```python
from build123d import *

# Parameters (mm, degrees)
SKETCH1_R           = 7.5
BOSS_EXTRUDE1_DEPTH = 56
CUT_EXTRUDE1_DEPTH  = 38
SKETCH3_R           = 7
CUT_EXTRUDE2_DEPTH  = 26


with BuildPart() as part:
    # Sketch1 → Boss-Extrude1 (new body)
    with BuildSketch(Plane.XY):
        with BuildLine():
            Line((-28, -19), (31, -19))
            Line((31, -19), (46, -10.339745962))
            Line((46, -10.339745962), (46, 10.339745962))
            Line((46, 10.339745962), (31, 19))
            Line((31, 19), (6.698703146, 19))
            ThreePointArc((6.698703146, 19), (-12.009583788, 15.368092477), (-28, 5))
            Line((-28, 5), (-28, -19))
        make_face()
        Circle(SKETCH1_R, mode=Mode.SUBTRACT)
    extrude(amount=BOSS_EXTRUDE1_DEPTH)

    # Sketch2 → Cut-Extrude1 (cut)
    with BuildSketch(Plane(origin=(0, 19, 0), x_dir=(1, 0, 0), z_dir=(0, 1, 0))):
        Polygon((31, 0), (46, -15), (46, 0), align=None)
        Polygon((31, -56), (46, -41), (46, -56), align=None)
        Polygon((-28, -8), (-12, -8), (-12, -14), (20, -14), (20, -42), (-12, -42), (-12, -48), (-28, -48), align=None)
    extrude(amount=-CUT_EXTRUDE1_DEPTH, mode=Mode.SUBTRACT)

    # Sketch3 → Cut-Extrude2 (cut)
    with BuildSketch(Plane(origin=(46, 0, 0), x_dir=(0, 0, -1), z_dir=(1, 0, 0))):
        with Locations((-28, 0)):
            Circle(SKETCH3_R)
    extrude(amount=-CUT_EXTRUDE2_DEPTH, mode=Mode.SUBTRACT)


solid = part.part
```
Check sheet for the modelled part. Datum: model origin and axes. Units: mm. A direction names the side the tool comes from. Give positions to 0.01 mm unless a question says otherwise; leave off trailing zeros. Order: outer loops, then holes, each group sorted by start corner. A loop starts at its lowest first (then second) coordinate and runs counter-clockwise, first axis right, second up. Notation, with made-up numbers: (47, 36.25) -> (103, 36.25) arc R25 cw to (103, 61.25) -> close; hole circle Ø8 at (27.25, 66.5). An arc over 180 degrees is marked (long way). Return JSON: item names as keys, results as strings.
1. Cross-section at C-C, the plane y = 0. Record the cut outline in (x, z), plus the area to 3 significant figures.
From the geometry:
{"outline": "(-28, 0) -> (-7.5, 0) -> (-7.5, 14) -> (-12, 14) -> (-12, 8) -> (-28, 8) -> close; (-28, 48) -> (-12, 48) -> (-12, 42) -> (-7.5, 42) -> (-7.5, 56) -> (-28, 56) -> close; (7.5, 0) -> (31, 0) -> (46, 15) -> (46, 21) -> (20, 21) -> (20, 14) -> (7.5, 14) -> close; (7.5, 42) -> (20, 42) -> (20, 35) -> (46, 35) -> (46, 41) -> (31, 56) -> (7.5, 56) -> close", "area": "1,600 mm^2"}
2. Cross-section at A-A, the plane z = 28. Record the cut outline in (x, y), plus the area to 3 significant figures.
From the geometry:
{"outline": "(20, -19) -> (31, -19) -> (46, -10.34) -> (46, -7) -> (20, -7) -> close; (20, 7) -> (46, 7) -> (46, 10.34) -> (31, 19) -> (20, 19) -> close", "area": "494 mm^2"}
3. Mould release check, pull along X, two halves, no side actions. Record for faces 3 (the cylindrical face through (-7.493, 0.33, 48.902)), 4 (the flat face through (46, -5, 34)), 5 (the flat face through (-28, -7, 52)), 6 (the flat face through (-20, -5, 48)): +X half, -X half, draft (parallel to the pull), parting line (faces both ways), or undercut.
From the geometry:
{"face 3": "undercut", "face 4": "+X half", "face 5": "-X half", "face 6": "draft"}
4. Set-up check for faces 1 (the flat face through (36.94, 15.57, 27.61)), 2 (the flat face through (20, 4, 22)): record each of +Z, -Z, +X, -X, +Y, -Y from which the full face is reachable in a straight line by a thin tool's end or side.
From the geometry:
{"face 1": "+Z, -Z, +X, +Y", "face 2": "-X, +Y, -Y"}
5. Go/stop test with flat-tipped pins: P1, Ø1.8, axis at y = 0, z = 46, coming from the -X side; P2, Ø12, axis at x = 37.5, y = 9.5, coming from the +Z side; P3, Ø1.5, axis at x = 18.5, z = 21, coming from the -Y side; P4, Ø8.5, axis at y = -5, z = 23, coming from the -X side. Record where each tip stops, or that it passes through.
From the geometry:
{"P1": "x = -12", "P2": "z = 55.5", "P3": "through", "P4": "x = 20"}
6. Cross-section at B-B, the plane x = 12. Record the cut outline in (y, z), plus the area to 3 significant figures.
From the geometry:
{"outline": "(-19, 0) -> (19, 0) -> (19, 14) -> (-19, 14) -> close; (-19, 42) -> (19, 42) -> (19, 56) -> (-19, 56) -> close", "area": "1,060 mm^2"}
7. Cross-section at D-D, the plane x = 0. Record the cut outline in (y, z).
From the geometry:
{"outline": "(-19, 0) -> (-7.5, 0) -> (-7.5, 14) -> (-19, 14) -> close; (-19, 42) -> (-7.5, 42) -> (-7.5, 56) -> (-19, 56) -> close; (7.5, 0) -> (18.55, 0) -> (18.55, 14) -> (7.5, 14) -> close; (7.5, 42) -> (18.55, 42) -> (18.55, 56) -> (7.5, 56) -> close"}
8. Material ranges on probe 1 along Z at (x, y) = (16, -4.5); probe 2 along Y at (x, z) = (27.5, 27.5); probe 3 along X at (y, z) = (-10, 16), recorded low to high. Write a range as [from, to].
From the geometry:
{"probe 1": "[0, 14], [42, 56]", "probe 2": "[-19, -6.98], [6.98, 19]", "probe 3": "[20, 46]"}
